Autodesk Fusion 360 part; units mm, degrees
sketch "Front-OuterDimensionsAndHoles" plane through (0, 0, 0) normal (0, 1, 0) x (1, 0, 0) in component "1006351A-GASKET"
  line L0 (-137.0277, -51.6717) -> (147.7462, -51.6717) construction
  line L1 (-113.1932, -37.4477) -> (126.9355, -37.4477) construction
  line L2 (-111.6736, 46.3723) -> (88.9542, 46.3723) construction
  line L3 (-83.38, 4.4623) -> (113.9408, 4.4623) construction
  line L4 (77.012, -30.3357) -> (138.7437, -30.3357) construction
  line L5 (77.3795, 43.3243) -> (102.1824, 43.3243) construction
  line L6 (-79.2352, -152.4901) -> (-79.2352, 67.7682) construction
  line L7 (80.7848, -152.4901) -> (80.7848, 99.4049) construction
  line L8 (-16.2432, -127.3246) -> (-16.2432, -37.4477) construction
  line L9 (-61.4552, -139.7875) -> (-61.4552, -23.5467) construction
  line L10 (-4.5592, -114.8617) -> (-4.5592, -39.3651) construction
  line L11 (0.7748, -102.6384) -> (0.7748, 79.7518) construction
  line L12 (6.1088, -89.6961) -> (6.1088, 17.4372) construction
  line L13 (122.5447, -1.8877) -> (-114.7303, -1.8877) construction
  line L14 (151.0657, 56.0243) -> (-121.6808, 56.0243) construction
  line L15 (-84.366, -162.1054) -> (-84.366, 89.1529) construction
  line L16 (84.8488, -151.7017) -> (84.8488, 106.4269) construction
  line L17 (17.7928, -77.6983) -> (17.7928, -42.3651) construction
  line L18 (63.0048, -65.3317) -> (63.0048, -43.9355) construction
  line L19 (-137.1695, 60.5963) -> (174.7441, 60.5963) construction
  line L20 (-87.8994, -47.0997) -> (156.6849, -47.0997) construction
  line L21 (70.6248, 70.8097) -> (70.6248, -45.2683) construction
  line L22 (16.2688, 71.2679) -> (16.2688, -42.3651) construction
  line L23 (-14.7192, 70.5042) -> (-14.7192, -42.9773) construction
  line L24 (-69.0752, 108.0768) -> (-69.0752, -44.9628) construction
  line L25 (-10.7822, 93.2616) -> (-10.7822, -44.6574) construction
  line L26 (73.9383, 85.014) -> (73.9383, -42.8245) construction
  line L27 (-101.4005, 49.5796) -> (76.5348, 49.5796) construction
  line L28 (-100.0259, -41.454) -> (76.8403, -41.454) construction
  line L29 (-78.8288, -51.9257) -> (79.3116, -51.9257)
  line L30 (84.8488, -46.3885) -> (84.8488, 54.8051)
  line L31 (79.3116, 60.3423) -> (-78.8288, 60.3423)
  line L32 (-84.366, 54.8051) -> (-84.366, -46.3885)
  line L33 (-65.9535, -37.7017) -> (-17.8829, -37.7017)
  line L34 (-14.7079, -34.5267) -> (-14.7079, 43.1257)
  line L35 (-17.8829, 46.3007) -> (-65.9535, 46.3007)
  line L36 (-69.1285, 43.1257) -> (-69.1285, -34.5267)
  line L37 (19.4438, -37.7017) -> (67.4498, -37.7017)
  line L38 (70.6248, -34.5267) -> (70.6248, 43.1585)
  line L39 (67.4498, 46.3335) -> (19.4438, 46.3335)
  line L40 (16.2688, 43.1585) -> (16.2688, -34.5267)
  arc A0 (-84.366, -46.3885) -> (-78.8288, -51.9257) centre (-78.8288, -46.3885) ccw
  arc A1 (-78.8288, 60.3423) -> (-84.366, 54.8051) centre (-78.8288, 54.8051) ccw
  arc A2 (84.8488, 54.8051) -> (79.3116, 60.3423) centre (79.3116, 54.8051) ccw
  arc A3 (-69.1285, -34.5267) -> (-65.9535, -37.7017) centre (-65.9535, -34.5267) ccw
  arc A4 (-17.8829, -37.7017) -> (-14.7079, -34.5267) centre (-17.8829, -34.5267) ccw
  arc A5 (-14.7079, 43.1257) -> (-17.8829, 46.3007) centre (-17.8829, 43.1257) ccw
  arc A6 (-65.9535, 46.3007) -> (-69.1285, 43.1257) centre (-65.9535, 43.1257) ccw
  arc A7 (67.4498, -37.7017) -> (70.6248, -34.5267) centre (67.4498, -34.5267) ccw
  arc A8 (70.6248, 43.1585) -> (67.4498, 46.3335) centre (67.4498, 43.1585) ccw
  arc A9 (19.4438, 46.3335) -> (16.2688, 43.1585) centre (19.4438, 43.1585) ccw
  arc A10 (16.2688, -34.5267) -> (19.4438, -37.7017) centre (19.4438, -34.5267) ccw
  arc A11 (79.3116, -51.9257) -> (84.8488, -46.3885) centre (79.3116, -46.3885) ccw
  line L41 (-100.3246, -43.4352) -> (86.6573, -43.4352) construction
  line L42 (-99.9078, -39.4728) -> (77.154, -39.4728) construction
  line L43 (-94.8446, 47.5984) -> (76.1721, 47.5984) construction
  line L44 (-94.4522, 51.5608) -> (76.1721, 51.5608) construction
  line L45 (-73.0122, 86.7279) -> (-73.0122, -45.4577) construction
  line L46 (-8.801, 72.5566) -> (-8.801, -44.6167) construction
  line L47 (-12.7634, 72.2199) -> (-12.7634, -44.6167) construction
  line L48 (-74.9934, 70.9572) -> (-74.9934, -44.6167) construction
  line L49 (-71.031, 71.0414) -> (-71.031, -44.3641) construction
  line L50 (-66.967, 51.5608) -> (-17.0814, 51.5608)
  line L51 (-8.928, 43.4074) -> (-8.928, -35.2818)
  line L52 (-17.0814, -43.4352) -> (-66.967, -43.4352)
  line L53 (-75.1204, -35.2818) -> (-75.1204, 43.4074)
  line L54 (-66.205, 47.5984) -> (-17.8434, 47.5984)
  line L55 (-12.8904, 42.6454) -> (-12.8904, -34.5198)
  line L56 (-17.8434, -39.4728) -> (-66.205, -39.4728)
  line L57 (-71.158, -34.5198) -> (-71.158, 42.6454)
  arc A12 (-75.1204, -35.2818) -> (-66.967, -43.4352) centre (-66.967, -35.2818) ccw
  arc A13 (-17.0814, -43.4352) -> (-8.928, -35.2818) centre (-17.0814, -35.2818) ccw
  arc A14 (-8.928, 43.4074) -> (-17.0814, 51.5608) centre (-17.0814, 43.4074) ccw
  arc A15 (-66.967, 51.5608) -> (-75.1204, 43.4074) centre (-66.967, 43.4074) ccw
  arc A16 (-71.158, -34.5198) -> (-66.205, -39.4728) centre (-66.205, -34.5198) ccw
  arc A17 (-66.205, 47.5984) -> (-71.158, 42.6454) centre (-66.205, 42.6454) ccw
  arc A18 (-12.8904, 42.6454) -> (-17.8434, 47.5984) centre (-17.8434, 42.6454) ccw
  arc A19 (-17.8434, -39.4728) -> (-12.8904, -34.5198) centre (-17.8434, -34.5198) ccw
  line L58 (18.631, -43.4352) -> (68.5166, -43.4352)
  arc A20 (68.5166, -43.4352) -> (76.67, -35.2818) centre (68.5166, -35.2818) ccw
  line L59 (76.67, -35.2818) -> (76.67, 43.4074)
  arc A21 (76.67, 43.4074) -> (68.5166, 51.5608) centre (68.5166, 43.4074) ccw
  line L60 (68.5166, 51.5608) -> (18.631, 51.5608)
  arc A22 (18.631, 51.5608) -> (10.4776, 43.4074) centre (18.631, 43.4074) ccw
  line L61 (10.4776, 43.4074) -> (10.4776, -35.2818)
  arc A23 (10.4776, -35.2818) -> (18.631, -43.4352) centre (18.631, -35.2818) ccw
  line L62 (19.393, -39.4728) -> (67.7546, -39.4728)
  arc A24 (67.7546, -39.4728) -> (72.7076, -34.5198) centre (67.7546, -34.5198) ccw
  line L63 (72.7076, -34.5198) -> (72.7076, 42.6454)
  arc A25 (72.7076, 42.6454) -> (67.7546, 47.5984) centre (67.7546, 42.6454) ccw
  line L64 (67.7546, 47.5984) -> (19.393, 47.5984)
  arc A26 (19.393, 47.5984) -> (14.44, 42.6454) centre (19.393, 42.6454) ccw
  line L65 (14.44, 42.6454) -> (14.44, -34.5198)
  line L66 (101.4573, -39.4728) -> (-75.6045, -39.4728) construction
  arc A27 (14.44, -34.5198) -> (19.393, -39.4728) centre (19.393, -34.5198) ccw
  point P0 (-79.2352, -47.0997)
  point P1 (-4.5592, -47.0997)
  point P2 (6.1088, -47.0997)
  point P3 (80.7848, -47.0997)
  point P4 (80.7848, 4.4623)
  point P5 (6.1088, 4.4623)
  point P6 (-79.2352, 4.4623)
  point P7 (-4.5592, 4.4623)
  point P8 (80.7848, 56.0243)
  point P9 (6.1088, 56.0243)
  point P10 (-4.5592, 56.0243)
  point P11 (-79.2352, 56.0243)
  point P12 (80.7848, -30.3357)
  point P13 (80.7848, 43.3243)
  point P14 (63.0048, -47.0997)
  point P15 (17.7928, -47.0997)
  point P16 (17.7928, 56.0243)
  point P17 (63.0048, 56.0243)
  point P18 (0.7748, -1.8877)
  point P19 (-16.2432, -47.0997)
  point P20 (-61.4552, -47.0997)
  point P21 (-79.2352, -30.3357)
  point P22 (-79.2352, 43.3243)
  point P23 (-61.4552, 56.0243)
  point P24 (-16.2432, 56.0243)
  dimension "d1" = 169.2148
  dimension "d2" = 4.064
  dimension "d3" = 160.02
  dimension "d4" = 142.24
  dimension "d5" = 97.028
  dimension "d6" = 85.344
  dimension "d7" = 80.01
  dimension "d8" = 74.676
  dimension "d9" = 17.78
  dimension "d10" = 62.992
  dimension "d12" = 112.268
  dimension "d13" = 103.124
  dimension "d14" = 51.562
  dimension "d16" = 57.912
  dimension "d17" = 86.36
  dimension "d18" = 12.7
  dimension "d19" = 14.224
  dimension "d20" = 4.572
  dimension "d21" = 14.224
  dimension "d22" = 14.224
  dimension "d23" = 54.356
  dimension "d24" = 54.356
  dimension "d25" = 91.0336
  dimension "d27" = 5.5372
  dimension "d28" = 5.5372
  dimension "d29" = 5.5372
  dimension "d30" = 3.175
  dimension "d31" = 3.175
  dimension "d32" = 3.175
  dimension "d33" = 3.175
  dimension "d34" = 3.175
  dimension "d35" = 3.175
  dimension "d36" = 3.175
  dimension "d37" = 3.175
  dimension "d40" = 5.5372
  dimension "d49" = 1.9812
  dimension "d50" = 1.9812
  dimension "d51" = 1.9812
  dimension "d52" = 1.9812
  dimension "d53" = 91.567
  dimension "d54" = 62.23
  dimension "d55" = 1.9812
  dimension "d56" = 1.9812
  dimension "d57" = 1.9812
  dimension "d58" = 1.9812
  dimension "d59" = 8.1534
  dimension "d60" = 8.1534
  dimension "d61" = 8.1534
  dimension "d62" = 8.1534
  dimension "d63" = 4.953
  dimension "d64" = 4.953
  dimension "d65" = 4.953
  dimension "d66" = 4.953
  dimension "d69" = 153.924
extrude "Extrude1" add sketch "Front-OuterDimensionsAndHoles" along normal blind 3.2004 contours L29 L30 L31 L32 A0 A1 A2 A11 | L50 L51 L52 L53 A12 A13 A14 A15 | L54 L55 L56 L57 A16 A17 A18 A19 | L58 A20 L59 A21 L60 A22 L61 A23 | L62 A24 L63 A25 L64 A26 L65 A27 in component "1006351A-GASKET"
hole "Hole1" at (80.7848, 0, 47.0997) at (6.1088, 0, 47.0997) at (-4.5592, 0, 47.0997) at (-79.2352, 0, 47.0997) at (-79.2352, 0, -56.0243) at (6.1088, 0, -56.0243) at (-4.5592, 0, -56.0243) at (80.7848, 0, -56.0243) at (80.7848, 0, -4.4623) at (6.1088, 0, -4.4623) at (-4.5592, 0, -4.4623) at (-79.2352, 0, -4.4623) direction (0, 1, 0) diameter 4.572 end through all in component "1006351A-GASKET"
hole "Hole2" at (-61.4552, 0, 47.0997) at (-16.2432, 0, 47.0997) at (17.7928, 0, 47.0997) at (63.0048, 0, 47.0997) at (80.7848, 0, 30.3357) at (80.7848, 0, -43.3243) at (63.0048, 0, -56.0243) at (0.7748, 0, 1.8877) at (-16.2432, 0, -56.0243) at (17.7928, 0, -56.0243) at (-61.4552, 0, -56.0243) at (-79.2352, 0, -43.3243) at (-79.2352, 0, 30.3357) direction (0, 1, 0) diameter 3.3782 end through all countersink diameter 5.842 countersink angle 82 in component "1006351A-GASKET"
extrude "Extrude2" cut sketch "Front-OuterDimensionsAndHoles" along normal blind 0.6604 contours L50 L51 L52 L53 A12 A13 A14 A15 | L58 A20 L59 A21 L60 A22 L61 A23 in component "1006351A-GASKET"
component "1006351A-GASKET" placed x (1, 0, 0) y (0, 1, 0) z (0, 0, 1) at (0, 0, 0)
equation "d49 = ( 0.156 / 2 ) * 1 in"
equation "d50 = ( 0.156 / 2 ) * 1 in"
equation "d51 = ( 0.156 / 2 ) * 1 in"
equation "d52 = ( 0.156 / 2 ) * 1 in"
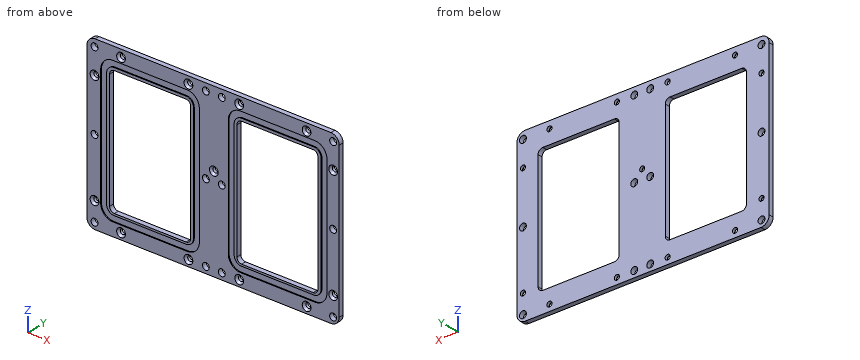
Can you work these out from the model? Positions are in its coordinate system, mm. Coordinates: 2 decimals unless noted, no trailing zeros. Loops run counter-clockwise (first coordinate to the right, second up) from the corner with the lowest first, then second, coordinate; pieces in that order, holes last. Notation, with made-up numbers: M -27.5,-14.5 L 31.5,-14.5 A9 cw 31.5,-6.5 Z; hole C 9,31.5 d2. An arc over 180 degrees is marked long. Answer as CSV lines item,"result". Start each with the question number.
1. Suppose I cut it at D-D, the plane y = 2.7. Count the separate pieces of the cut face and the enclosed holes in it, plus the area to 3 significant figures.
2. Suppose I cut it at C-C, the plane x = -51. List the corners of the cut face in (y, z) for me.
3. If I drill on probe 1 along X at (y, z) = (2.55, -12); probe 2 along Z at (x, y) = (36.5, 2.55); probe 3 along Z at (x, y) = (37, 0.3), over which ranges is the centre line in solid material (lowest first)? Write a range as [from, to].
4. Suppose I cut it at B-B, the plane x = 27.5. List the corners of the cut face in (y, z) for me.
5. Suppose I cut it at A-A, the plane z = -15. List the corners of the cut face in (x, y) for me.
Output:
1,separate pieces,"1"
1,enclosed holes,"27"
1,area,"9,540 mm^2"
2,outline,"M 0,-60.34 L 3.2,-60.34 L 3.2,-46.3 L 0,-46.3 L 0,-47.6 L 0.66,-47.6 L 0.66,-51.56 L 0,-51.56 Z; M 0,37.7 L 3.2,37.7 L 3.2,51.93 L 0,51.93 L 0,43.44 L 0.66,43.44 L 0.66,39.47 L 0,39.47 Z"
3,probe 1,"x = [-84.37, -69.13], [-14.71, 16.27], [70.62, 84.85]"
3,probe 2,"z = [-60.34, -46.33], [37.7, 51.93]"
3,probe 3,"z = [-60.34, -51.56], [-47.6, -46.33], [37.7, 39.47], [43.44, 51.93]"
4,outline,"M 0,-60.34 L 3.2,-60.34 L 3.2,-46.33 L 0,-46.33 L 0,-47.6 L 0.66,-47.6 L 0.66,-51.56 L 0,-51.56 Z; M 0,37.7 L 3.2,37.7 L 3.2,51.93 L 0,51.93 L 0,43.44 L 0.66,43.44 L 0.66,39.47 L 0,39.47 Z"
5,outline,"M -84.37,0 L -75.12,0 L -75.12,0.66 L -71.16,0.66 L -71.16,0 L -69.13,0 L -69.13,3.2 L -84.37,3.2 Z; M -14.71,0 L -12.89,0 L -12.89,0.66 L -8.93,0.66 L -8.93,0 L 10.48,0 L 10.48,0.66 L 14.44,0.66 L 14.44,0 L 16.27,0 L 16.27,3.2 L -14.71,3.2 Z; M 70.62,0 L 72.71,0 L 72.71,0.66 L 76.67,0.66 L 76.67,0 L 84.85,0 L 84.85,3.2 L 70.62,3.2 Z"
